Part model, mm, in its own coordinate system. Face numbers are marked on the shaded views. A direction names the side the tool comes from. Coordinates: 2 decimals unless noted, no trailing zeros. Write each loop counter-clockwise with the first axis right and the second up, starting at its lowest first coordinate (ties: lowest second). Pieces come first, ordered by that corner, then holes. Notation, with made-up numbers: (27.5, -29.75) - (47.5, -29.75) arc R26 ccw to (47.5, 1.25) - close; hole circle Ø2 at (68, 78). An arc over 180 degrees is marked (long way). Write each question's results on one line, items separated by ' | '.
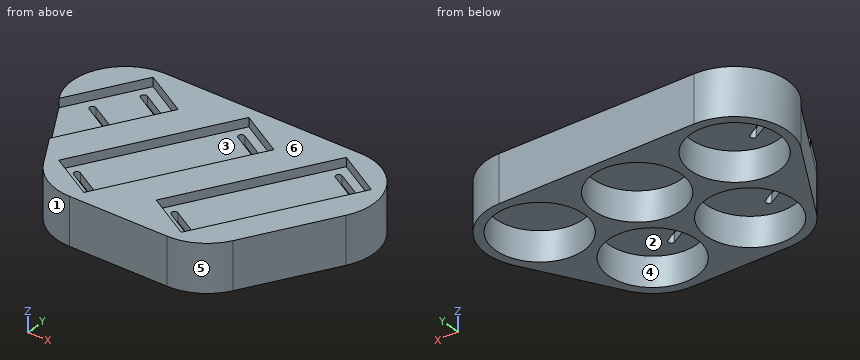
from build123d import *

# Parameters (mm, degrees)
SKETCH1_R           = 7.5
BOSS_EXTRUDE1_DEPTH = 5
SKETCH2_R           = 7.5
BOSS_EXTRUDE2_DEPTH = 1.5
BOSS_EXTRUDE3_DEPTH = 1.5


with BuildPart() as part:
    # Sketch1 → Boss-Extrude1 (new body)
    with BuildSketch(Plane.XY):
        with BuildLine():
            Line((7.794228634, -4.5), (-0.455771366, -18.789419162))
            ThreePointArc((-0.455771366, -18.789419162), (-3.75, -22.083647797), (-8.25, -23.289419162))
            Line((-8.25, -23.289419162), (-24.75, -23.289419162))
            ThreePointArc((-24.75, -23.289419162), (-29.25, -22.083647797), (-32.544228634, -18.789419162))
            Line((-32.544228634, -18.789419162), (-40.794228634, -4.5))
            ThreePointArc((-40.794228634, -4.5), (-40.794228634, 4.5), (-33, 9))
            Line((-33, 9), (0, 9))
            ThreePointArc((0, 9), (7.794228634, 4.5), (7.794228634, -4.5))
        make_face()
        with Locations((-24.75, -14.289419162)):
            Circle(SKETCH1_R, mode=Mode.SUBTRACT)
        with Locations((-16.5, 0)):
            Circle(SKETCH1_R, mode=Mode.SUBTRACT)
        Circle(SKETCH1_R, mode=Mode.SUBTRACT)
        with Locations((-8.25, -14.289419162)):
            Circle(SKETCH1_R, mode=Mode.SUBTRACT)
        with Locations((-33, 0)):
            Circle(SKETCH1_R, mode=Mode.SUBTRACT)
    extrude(amount=BOSS_EXTRUDE1_DEPTH)

    # Sketch2 → Boss-Extrude2 (add)
    # profile 1 of 6: a face of its own
    with BuildSketch(Plane.XY.offset(5)):
        with BuildLine():
            Line((-0.455771366, -18.789419162), (7.794228634, -4.5))
            ThreePointArc((7.794228634, -4.5), (7.794228634, 4.5), (0, 9))
            Line((0, 9), (-33, 9))
            ThreePointArc((-33, 9), (-40.794228634, 4.5), (-40.794228634, -4.5))
            Line((-40.794228634, -4.5), (-32.544228634, -18.789419162))
            ThreePointArc((-32.544228634, -18.789419162), (-29.25, -22.083647797), (-24.75, -23.289419162))
            Line((-24.75, -23.289419162), (-8.25, -23.289419162))
            ThreePointArc((-8.25, -23.289419162), (-3.75, -22.083647797), (-0.455771366, -18.789419162))
        make_face()
        Circle(SKETCH2_R, mode=Mode.SUBTRACT)
        with Locations((-16.5, 0)):
            Circle(SKETCH2_R, mode=Mode.SUBTRACT)
        with Locations((-33, 0)):
            Circle(SKETCH2_R, mode=Mode.SUBTRACT)
        with Locations((-24.75, -14.289419162)):
            Circle(SKETCH2_R, mode=Mode.SUBTRACT)
        with Locations((-8.25, -14.289419162)):
            Circle(SKETCH2_R, mode=Mode.SUBTRACT)
    # profile 2 of 6: a face of its own
    with BuildSketch(Plane.XY.offset(5)):
        with Locations((-8.25, -14.289419162)):
            Circle(SKETCH2_R)
        with BuildLine():
            ThreePointArc((-12.040063509, -15.854001725), (-12.723076211, -16.037014427), (-12.540063509, -16.720027129))
            Line((-12.540063509, -16.720027129), (-8.209936491, -19.220027129))
            ThreePointArc((-8.209936491, -19.220027129), (-7.526923789, -19.037014427), (-7.709936491, -18.354001725))
            Line((-7.709936491, -18.354001725), (-12.040063509, -15.854001725))
        make_face(mode=Mode.SUBTRACT)
    # profile 3 of 6: a face of its own
    with BuildSketch(Plane.XY.offset(5)):
        Circle(SKETCH2_R)
        with BuildLine():
            ThreePointArc((-0.040063509, 4.930607966), (-0.723076211, 4.747595264), (-0.540063509, 4.064582562))
            Line((-0.540063509, 4.064582562), (3.790063509, 1.564582562))
            ThreePointArc((3.790063509, 1.564582562), (4.473076211, 1.747595264), (4.290063509, 2.430607966))
            Line((4.290063509, 2.430607966), (-0.040063509, 4.930607966))
        make_face(mode=Mode.SUBTRACT)
    # profile 4 of 6: a face of its own
    with BuildSketch(Plane.XY.offset(5)):
        with Locations((-16.5, 0)):
            Circle(SKETCH2_R)
        with BuildLine():
            ThreePointArc((-16.540063509, 4.930607966), (-17.223076211, 4.747595264), (-17.040063509, 4.064582562))
            Line((-17.040063509, 4.064582562), (-12.709936491, 1.564582562))
            ThreePointArc((-12.709936491, 1.564582562), (-12.026923789, 1.747595264), (-12.209936491, 2.430607966))
            Line((-12.209936491, 2.430607966), (-16.540063509, 4.930607966))
        make_face(mode=Mode.SUBTRACT)
    # profile 5 of 6: a face of its own
    with BuildSketch(Plane.XY.offset(5)):
        with Locations((-24.75, -14.289419162)):
            Circle(SKETCH2_R)
        with BuildLine():
            ThreePointArc((-28.540063509, -15.854001725), (-29.223076211, -16.037014427), (-29.040063509, -16.720027129))
            Line((-29.040063509, -16.720027129), (-24.709936491, -19.220027129))
            ThreePointArc((-24.709936491, -19.220027129), (-24.026923789, -19.037014427), (-24.209936491, -18.354001725))
            Line((-24.209936491, -18.354001725), (-28.540063509, -15.854001725))
        make_face(mode=Mode.SUBTRACT)
    # profile 6 of 6: a face of its own
    with BuildSketch(Plane.XY.offset(5)):
        with Locations((-33, 0)):
            Circle(SKETCH2_R)
        with BuildLine():
            ThreePointArc((-36.790063509, -1.564582562), (-37.473076211, -1.747595264), (-37.290063509, -2.430607966))
            Line((-37.290063509, -2.430607966), (-32.959936491, -4.930607966))
            ThreePointArc((-32.959936491, -4.930607966), (-32.276923789, -4.747595264), (-32.459936491, -4.064582562))
            Line((-32.459936491, -4.064582562), (-36.790063509, -1.564582562))
        make_face(mode=Mode.SUBTRACT)
        with BuildLine():
            ThreePointArc((-33.040063509, 4.930607966), (-33.723076211, 4.747595264), (-33.540063509, 4.064582562))
            Line((-33.540063509, 4.064582562), (-29.209936491, 1.564582562))
            ThreePointArc((-29.209936491, 1.564582562), (-28.526923789, 1.747595264), (-28.709936491, 2.430607966))
            Line((-28.709936491, 2.430607966), (-33.040063509, 4.930607966))
        make_face(mode=Mode.SUBTRACT)
    extrude(amount=BOSS_EXTRUDE2_DEPTH)

    # Sketch3 → Boss-Extrude3 (add)
    with BuildSketch(Plane.XY.offset(6.5)):
        with BuildLine():
            ThreePointArc((-33, 9), (-40.794228634, 4.5), (-40.794228634, -4.5))
            Line((-40.794228634, -4.5), (-40.72205985, -4.625))
            Line((-40.72205985, -4.625), (-33.851361142, 7.275399247))
            Line((-33.851361142, 7.275399247), (-26.273638858, 2.900399247))
            Line((-26.273638858, 2.900399247), (-35.670244995, -13.375))
            Line((-35.670244995, -13.375), (-32.544228634, -18.789419162))
            ThreePointArc((-32.544228634, -18.789419162), (-29.25, -22.083647797), (-24.75, -23.289419162))
            Line((-24.75, -23.289419162), (-8.25, -23.289419162))
            ThreePointArc((-8.25, -23.289419162), (-3.75, -22.083647797), (-0.455771366, -18.789419162))
            Line((-0.455771366, -18.789419162), (7.794228634, -4.5))
            ThreePointArc((7.794228634, -4.5), (7.794228634, 4.5), (0, 9))
            Line((0, 9), (-33, 9))
        make_face()
        Polygon((-17.476361142, 7.058892896), (-9.898638858, 2.683892896), (-23.773638858, -21.348312059), (-31.351361142, -16.973312059), align=None, mode=Mode.SUBTRACT)
        Polygon((-0.976361142, 7.058892896), (6.601361142, 2.683892896), (-7.273638858, -21.348312059), (-14.851361142, -16.973312059), align=None, mode=Mode.SUBTRACT)
    extrude(amount=BOSS_EXTRUDE3_DEPTH)


solid = part.part
(1) Saw through at C-C on z = 3. Write the cut outline in (x, y).
Return value:
outline: (-40.79, -4.5) - (-32.54, -18.79) arc R9 ccw to (-24.75, -23.29) - (-8.25, -23.29) arc R9 ccw to (-0.46, -18.79) - (7.79, -4.5) arc R9 ccw to (0, 9) - (-33, 9) arc R9 ccw to start; hole circle Ø15 at (-33, 0); hole circle Ø15 at (-24.75, -14.29); hole circle Ø15 at (-16.5, 0); hole circle Ø15 at (-8.25, -14.29); hole circle Ø15 at (0, 0)
(2) Saw through at D-D on y = 0. Write the cut outline in (x, z), then the cut area to 3 significant figures.
Return value:
outline: (-42, 0) - (-40.5, 0) - (-40.5, 5) - (-25.5, 5) - (-25.5, 0) - (-24, 0) - (-24, 5) - (-9, 5) - (-9, 0) - (-7.5, 0) - (-7.5, 5) - (7.5, 5) - (7.5, 0) - (9, 0) - (9, 8) - (5.05, 8) - (5.05, 6.5) - (-5.05, 6.5) - (-5.05, 8) - (-11.45, 8) - (-11.45, 6.5) - (-21.55, 6.5) - (-21.55, 8) - (-27.95, 8) - (-27.95, 6.5) - (-38.05, 6.5) - (-38.05, 8) - (-42, 8) - close | area: 138 mm^2
(3) Wall check: line 1 (X direction, y = -20.5, z = 2.5); line 2 (Y direction, x = -19, z = 2.25); line 3 (X direction, y = -4, z = 1.75). Give the ranges that are in metal, low to high. Write a range as from..to.
Return value:
line 1: x = -31.26..-28.95, -20.55..-12.45, -4.05..-1.74 | line 2: y = -23.29..-19.1, -9.47..-7.07, 7.07..9 | line 3: x = -41.06..-39.34, -26.66..-22.84, -10.16..-6.34, 6.34..8.06
(4) Two-plate mould, pull along X, no slides. Class the marked faces 4, 5 and 6: released by +X, released by -X, zero draft, split by the parting line, or undercut.
Return value:
face 4: undercut | face 5: released by +X | face 6: zero draft
(5) Saw through at B-B on x = -20. Write the cut outline in (y, z).
Return value:
outline: (-23.29, 0) - (-20.09, 0) - (-20.09, 5) - (-8.49, 5) - (-8.49, 0) - (-6.63, 0) - (-6.63, 5) - (6.63, 5) - (6.63, 0) - (9, 0) - (9, 8) - (2.69, 8) - (2.69, 6.5) - (-14.81, 6.5) - (-14.81, 8) - (-23.29, 8) - close
(6) 3-axis set-ups, long thin cutter, end or side, ignore diameter. For the marked faces 1, 2 and 3: which of +Z, -Z, +X, -X, +Y, -Y reach the whole face in a straight line?
Return value:
face 1: +Z, -Z, -X, -Y | face 2: -Z | face 3: +Z
(7) Saw through at A-A on z = 5.75. Count the separate pieces of the cut face and the enclosed holes in it, then the cut area to 3 significant figures.
Return value:
separate pieces: 1 | enclosed holes: 6 | area: 1,320 mm^2
(8) Flat gauge pins, fed straight in: P1, Ø4, axis at y = 5, z = 2, coming from the +X side; P2, Ø4, axis at x = -0.5, z = 2.5, coming from the -Y side; P3, Ø7.5, axis at x = 1.5, y = 2.5, coming from the -Z side. Where does each tip first touch, or does it go through?
Return value:
P1: stops at x = 8.49 | P2: stops at y = -21.21 | P3: stops at z = 5
